For this review, take the finished solid that the model builds, in its own axes (mm). A direction names the side the tool comes from. Coordinates: 2 decimals unless noted, no trailing zeros. Write each loop counter-clockwise with the first axis right and the second up, starting at its lowest first coordinate (ties: lowest second). Pieces come first, ordered by that corner, then holes.
```python
from build123d import *

# Parameters (mm, degrees)
SKETCH1_W           = 130
SKETCH1_H           = 50
BOSS_EXTRUDE2_DEPTH = 6
SKETCH5_W           = 27
SKETCH5_H           = 50
BOSS_EXTRUDE4_DEPTH = 27
SKETCH6_R           = 11
CUT_EXTRUDE3_DEPTH  = 3.8
SKETCH8_R           = 5
CUT_EXTRUDE4_DEPTH  = 12
CUT_EXTRUDE5_START  = -3.8
SKETCH9_R           = 11
CUT_EXTRUDE5_DEPTH  = 3.8
CUT_EXTRUDE6_START  = -12.5
SKETCH10_R          = 5
CUT_EXTRUDE6_DEPTH  = 12.5
FILLET1_R           = 10
FILLET2_R           = 10
CUT_EXTRUDE7_START  = -90
SKETCH10_2_R        = 5
CUT_EXTRUDE7_DEPTH  = 90
SKETCH14_R          = 20
BOSS_EXTRUDE5_DEPTH = 20
SKETCH15_R          = 17.25
CUT_EXTRUDE8_DEPTH  = 60
SKETCH16_W          = 130
SKETCH16_H          = 50
CUT_EXTRUDE9_DEPTH  = 3


with BuildPart() as part:
    # Sketch1 → Boss-Extrude2 (new body)
    with BuildSketch(Plane(origin=(0, 0, 0), x_dir=(1, 0, 0), z_dir=(0, 1, 0))):
        Rectangle(SKETCH1_W, SKETCH1_H)
    extrude(amount=BOSS_EXTRUDE2_DEPTH)

    # Sketch5 → Boss-Extrude4 (add)
    with BuildSketch(Plane(origin=(0, 6, 0), x_dir=(1, 0, 0), z_dir=(0, 1, 0))):
        with Locations((51.5, 0)):
            Rectangle(SKETCH5_W, SKETCH5_H)
    extrude(amount=BOSS_EXTRUDE4_DEPTH)

    # Sketch6 → Cut-Extrude3 (cut)
    with BuildSketch(Plane.XY.offset(25)):
        with Locations((51.5, 19.5)):
            Circle(SKETCH6_R)
    extrude(amount=-CUT_EXTRUDE3_DEPTH, mode=Mode.SUBTRACT)

    # Sketch8 → Cut-Extrude4 (cut)
    with BuildSketch(Plane.XY.offset(21.2)):
        with Locations((51.5, 19.5)):
            Circle(SKETCH8_R)
    extrude(amount=-CUT_EXTRUDE4_DEPTH, mode=Mode.SUBTRACT)

    # Sketch9 → Cut-Extrude5 (cut)
    with BuildSketch(Plane(origin=(0, 0, -25), x_dir=(-1, 0, 0), z_dir=(0, 0, -1)).offset(CUT_EXTRUDE5_START)):
        with Locations(Location((-51.5, 19.5, 0), (0, 0, 180))):
            Circle(SKETCH9_R)
    extrude(amount=CUT_EXTRUDE5_DEPTH, mode=Mode.SUBTRACT)

    # Sketch10 → Cut-Extrude6 (cut)
    with BuildSketch(Plane(origin=(0, 0, -21.2), x_dir=(-1, 0, 0), z_dir=(0, 0, -1)).offset(CUT_EXTRUDE6_START)):
        with Locations(Location((-51.5, 19.5, 0), (0, 0, 180))):
            Circle(SKETCH10_R)
    extrude(amount=CUT_EXTRUDE6_DEPTH, mode=Mode.SUBTRACT)

    # Fillet1
    fillet1_edges = [part.edges().sort_by_distance(p)[0] for p in [
        (38, 33, 0),
    ]]
    fillet(fillet1_edges, radius=FILLET1_R)

    # Fillet2
    fillet2_edges = [part.edges().sort_by_distance(p)[0] for p in [
        (65, 33, 0),
    ]]
    fillet(fillet2_edges, radius=FILLET2_R)

    # Sketch10_2 → Cut-Extrude7 (cut)
    with BuildSketch(Plane(origin=(0, 0, -21.2), x_dir=(-1, 0, 0), z_dir=(0, 0, -1)).offset(CUT_EXTRUDE7_START)):
        with Locations(Location((-51.5, 19.5, 0), (0, 0, 180))):
            Circle(SKETCH10_2_R)
    extrude(amount=CUT_EXTRUDE7_DEPTH, mode=Mode.SUBTRACT)

    # Sketch14 → Boss-Extrude5 (add)
    with BuildSketch(Plane(origin=(0, 6, 0), x_dir=(1, 0, 0), z_dir=(0, 1, 0))):
        with Locations(Location((0, 0, 0), (0, 0, 270))):
            Circle(SKETCH14_R)
    extrude(amount=BOSS_EXTRUDE5_DEPTH)

    # Sketch15 → Cut-Extrude8 (cut)
    with BuildSketch(Plane(origin=(0, 26, 0), x_dir=(1, 0, 0), z_dir=(0, 1, 0))):
        with Locations(Location((0, 0, 0), (0, 0, 270))):
            Circle(SKETCH15_R)
    extrude(amount=-CUT_EXTRUDE8_DEPTH, mode=Mode.SUBTRACT)

    # Sketch16 → Cut-Extrude9 (cut)
    with BuildSketch(Plane.XZ):
        Rectangle(SKETCH16_W, SKETCH16_H)
    extrude(amount=-CUT_EXTRUDE9_DEPTH, mode=Mode.SUBTRACT)


solid = part.part
```
Q1. For probe 1 along Y at (x, z) = (51, 16); probe 2 along X at (y, z) = (14, 11.5); probe 3 along X at (y, z) = (10, 15.5), list the stretches that pass through material, from the lowest coordinate up.
Ans:
probe 1: y = 3 to 14.53, 24.47 to 33
probe 2: x = -16.36 to -12.86, 12.86 to 16.36, 38 to 65
probe 3: x = -12.64 to -7.57, 7.57 to 12.64, 38 to 65
Q2. Add section A-A (y = 19.5). State the section outline as (x, z) points.
Ans:
outline: circle Ø40 at (0, 0); (38, -25) - (40.5, -25) - (40.5, -21.2) - (46.5, -21.2) - (46.5, 21.2) - (40.5, 21.2) - (40.5, 25) - (38, 25) - close; (56.5, -21.2) - (62.5, -21.2) - (62.5, -25) - (65, -25) - (65, 25) - (62.5, 25) - (62.5, 21.2) - (56.5, 21.2) - close; hole circle Ø34.5 at (0, 0)
Q3. Add section B-B (z = 0). State the section outline as (x, y) points.
Ans:
outline: (-65, 3) - (-17.25, 3) - (-17.25, 26) - (-20, 26) - (-20, 6) - (-65, 6) - close; (17.25, 3) - (65, 3) - (65, 23) arc R10 ccw to (55, 33) - (48, 33) arc R10 ccw to (38, 23) - (38, 6) - (20, 6) - (20, 26) - (17.25, 26) - close; hole circle Ø10 at (51.5, 19.5)
Q4. Add section D-D (z = -18.5). State the section outline as (x, y) points, then the cut area to 3 significant figures.
Ans:
outline: (-65, 3) - (65, 3) - (65, 23) arc R10 ccw to (55, 33) - (48, 33) arc R10 ccw to (38, 23) - (38, 6) - (7.6, 6) - (7.6, 26) - (-7.6, 26) - (-7.6, 6) - (-65, 6) - close; hole circle Ø10 at (51.5, 19.5)
area: 1,300 mm2
Q5. Tool access review of faces 4 (the cylindrical face through (-19.524, 15.86, -4.336)), 5 (the flat face through (-9, 26, -15)), 6 (the cylindrical face through (40.85, 29.99, -0.35)), 7 (the flat face through (56.2, 17.2, 21.2)), 8 (the cylindrical face through (49.12, 30.24, -23.07)): name each direction out of +Z, -Z, +X, -X, +Y, -Y from which nothing blocks a thin tool from reaching the whole face with its end or side.
Ans:
face 4: +Y
face 5: +Z, -Z, -X, +Y
face 6: +Z, -Z, +Y
face 7: +Z
face 8: -Z
Q6. Add section C-C (x = 51.5). State the section outline as (y, z) points.
Ans:
outline: (3, -25) - (8.5, -25) - (8.5, -21.2) - (14.5, -21.2) - (14.5, 21.2) - (8.5, 21.2) - (8.5, 25) - (3, 25) - close; (24.5, -21.2) - (30.5, -21.2) - (30.5, -25) - (33, -25) - (33, 25) - (30.5, 25) - (30.5, 21.2) - (24.5, 21.2) - close
Q7. Clearance check with flat-ended pins moving along their axes: pin 1 Ø8.5 at (y, z) = (13, 1) entering from -X; pin 2 Ø15 at (x, z) = (-11, 3) entering from +Y; pin 3 Ø13 at (x, y) = (51.5, 19.5) entering from -Z; pin 4 Ø17.5 at (x, y) = (46.5, 16.5) entering from -Z. State where each tip first meets the part, or that it passes through.
Ans:
pin 1: stops at x = -20
pin 2: stops at y = 26
pin 3: stops at z = -21.2
pin 4: stops at z = -25
Q8. Draft analysis for pull direction Y (two halves, no side actions). For faces 1 (the flat face through (-15, 3, 11)), 2 (the flat face through (19, 5.7, 25)), 3 (the flat face through (56.2, 21.8, -21.2)), state which applies: +Y half, -Y half, draft (parallel to the pull), parting line (faces both ways), or undercut.
Ans:
face 1: -Y half
face 2: draft
face 3: undercut
